from build123d import *

# Parameters (mm, degrees)
SKETCH1_R           = 1.5
BOSS_EXTRUDE1_DEPTH = 3


with BuildPart() as part:
    # Sketch1 → Boss-Extrude1 (new body)
    with BuildSketch(Plane(origin=(0, 0, 0), x_dir=(1, 0, 0), z_dir=(0, 1, 0))):
        with BuildLine():
            Line((-11.129677419, 1.625806452), (7.870322581, 1.625806452))
            ThreePointArc((7.870322581, 1.625806452), (9.284536143, 1.040020014), (9.870322581, -0.374193548))
            Line((9.870322581, -0.374193548), (9.870322581, -7.374193548))
            Line((9.870322581, -7.374193548), (3.370322581, -7.374193548))
            Line((3.370322581, -7.374193548), (3.370322581, -10.374193548))
            Line((3.370322581, -10.374193548), (-6.629677419, -10.374193548))
            Line((-6.629677419, -10.374193548), (-6.629677419, -7.374193548))
            Line((-6.629677419, -7.374193548), (-13.129677419, -7.374193548))
            Line((-13.129677419, -7.374193548), (-13.129677419, -0.374193548))
            ThreePointArc((-13.129677419, -0.374193548), (-12.543890982, 1.040020014), (-11.129677419, 1.625806452))
        make_face()
        with Locations((-4.629677419, -2.374193548)):
            Circle(SKETCH1_R, mode=Mode.SUBTRACT)
        with Locations((1.370322581, -2.374193548)):
            Circle(SKETCH1_R, mode=Mode.SUBTRACT)
    extrude(amount=BOSS_EXTRUDE1_DEPTH)


solid = part.part
The listing builds one solid part. Answer for the finished solid, in the listing's coordinates (mm). A direction names the side the tool comes from. Give positions to 0.01 mm unless a question says otherwise; leave off trailing zeros. Write each loop counter-clockwise with the first axis right and the second up, starting at its lowest first coordinate (ties: lowest second). Pieces come first, ordered by that corner, then holes. Notation, with made-up numbers: (52.25, -4.5) - (72.25, -4.5) arc R12 ccw to (72.25, 6.5) - close; hole circle Ø3 at (-35, 81.5). An arc over 180 degrees is marked (long way). One line per question, with ' | ' between items. Start each with the question number.
1. Given P1, Ø0.9, axis at x = -10.5, y = 1.5, coming from the +Z side; P2, Ø0.9, axis at y = 2, z = 8, coming from the -X side; P3, Ø0.9, axis at y = 1.5, z = 9, coming from the +X side, each flat-ended and moving along its own axis, determine where each tip first touches the part or whether it passes through.
2. For faces 5 (the face through (7, 1, 7.374)), 6 (the face through (-10, 1, 7.374)), 7 (the face through (9.87, 1, 4)), determine the directions among +Z, -Z, +X, -X, +Y, -Y from which every point of the face is accessible in a straight line to the end or side of a thin tool.
3. Section D-D, the plane x = 7.5 is taken. Determine the outline of the cut face in (y, z), then the cut area to 3 significant figures.
4. Section C-C, the plane z = 2 is taken. Determine the outline of the cut face in (x, y), then the cut area to 3 significant figures.
5. Section B-B, the plane y = 1.65 is taken. Determine the outline of the cut face in (x, z), then the cut area to 3 significant figures.
6. Straight lines are drawn through the part: line 1 (Z direction, x = -4.75, y = 0.2); line 2 (Z direction, x = -8, y = 2.45); line 3 (X direction, y = 0.5, z = 3.5). For each, find the intervals that lie inside material, in ascending order.
7. Determine the mould class of faces 1 (the face through (-6.63, 1, 9)), 2 (the face through (-2, 1, 10.374)), 3 (the face through (-12.559, 1.479, -1.024)), 4 (the face through (-3.244, 1.479, 2.949)) for opening direction Z: +Z half, -Z half, draft (parallel to the pull), parting line (faces both ways), or undercut.
8. Section A-A, the plane x = -4.75 is taken. Determine the outline of the cut face in (y, z), then the cut area to 3 significant figures.
Result:
1) P1: stops at z = 7.37 | P2: stops at x = -6.63 | P3: stops at x = 3.37
2) face 5: +Z, +X, +Y, -Y | face 6: +Z, -X, +Y, -Y | face 7: +Z, -Z, +X, +Y, -Y
3) outline: (0, -1.63) - (3, -1.63) - (3, 7.37) - (0, 7.37) - close | area: 27.0 mm2
4) outline: (-13.13, 0) - (-6.08, 0) - (-6.08, 3) - (-13.13, 3) - close; (-3.18, 0) - (-0.08, 0) - (-0.08, 3) - (-3.18, 3) - close; (2.82, 0) - (9.87, 0) - (9.87, 3) - (2.82, 3) - close | area: 51.6 mm2
5) outline: (-13.13, 0.37) arc R2 ccw to (-11.13, -1.63) - (7.87, -1.63) arc R2 ccw to (9.87, 0.37) - (9.87, 7.37) - (3.37, 7.37) - (3.37, 10.37) - (-6.63, 10.37) - (-6.63, 7.37) - (-13.13, 7.37) - close; hole circle Ø3 at (-4.63, 2.37); hole circle Ø3 at (1.37, 2.37) | area: 221 mm2
6) line 1: z = -1.63 to 0.88, 3.87 to 10.37 | line 2: z = -1.63 to 7.37 | line 3: x = -13.13 to -5.62, -3.64 to 0.38, 2.36 to 9.87
7) face 1: draft | face 2: +Z half | face 3: -Z half | face 4: undercut
8) outline: (0, -1.63) - (3, -1.63) - (3, 0.88) - (0, 0.88) - close; (0, 3.87) - (3, 3.87) - (3, 10.37) - (0, 10.37) - close | area: 27.0 mm2
